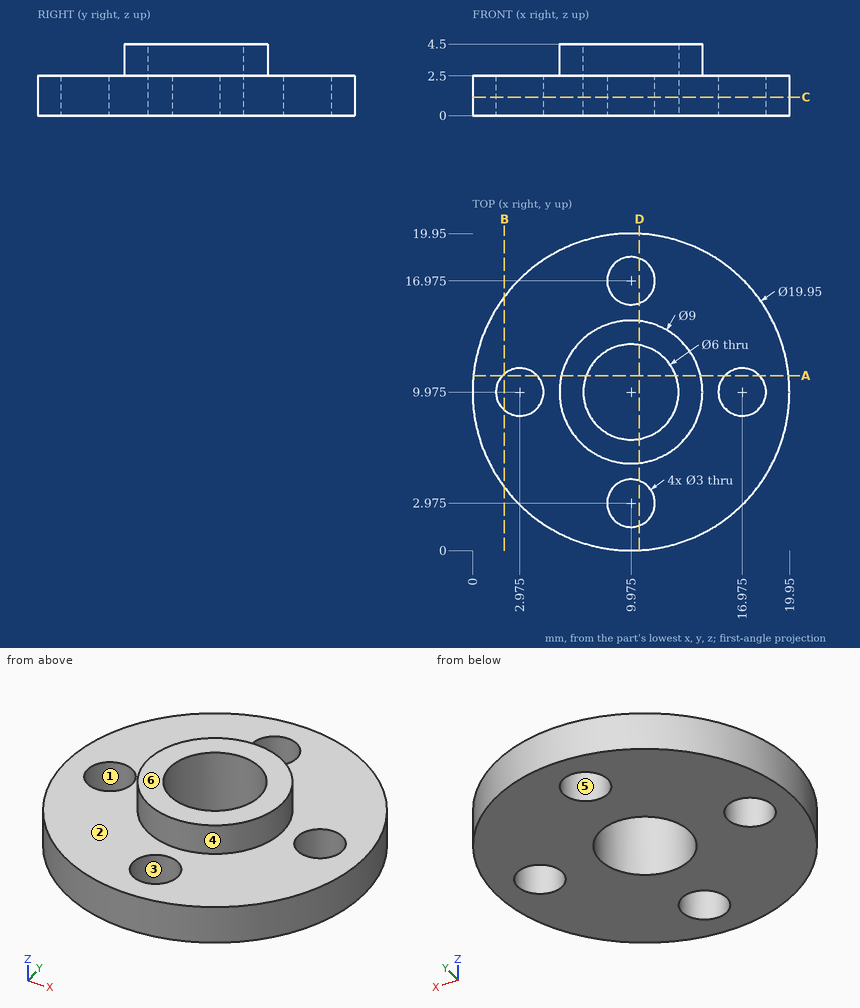
For this review, use the dimensioned drawing (mm, ordinates from the lowest corner) and the shaded views. A direction names the side the tool comes from. Coordinates: 2 decimals unless noted, no trailing zeros. Loops run counter-clockwise (first coordinate to the right, second up) from the corner with the lowest first, then second, coordinate; pieces in that order, holes last.
1. For line 1 (Y direction, x = 10.5, z = 2.15); line 2 (X direction, y = 11, z = 1.4); line 3 (Y direction, x = 9, z = 1.65), list the stretches that pass through material, from the lowest coordinate up.
2. Add section D-D, the plane x = 10.5. Give the boundary of the cut face in (y, z), then the cut area to 3 significant figures.
3. Add section B-B, the plane x = 2. Give the boundary of the cut face in (y, z).
4. Add section A-A, the plane y = 11. Give the boundary of the cut face in (x, z).
5. Mouldability with a two-part tool opening along X and no side actions: class the marked faces 3, 4, 5 and 6 as +X half, -X half, draft (parallel to the pull), parting line (faces both ways), or undercut.
6. Insertion check: P1, Ø1, axis at x = 7, z = 2, coming from the +Y side; P2, Ø4, axis at x = 16.975, y = 9.975, coming from the +Z side; P3, Ø2, axis at y = 8.5, z = 0.5, coming from the +X side; P4, Ø2.5, axis at x = 9.975, y = 2.975, coming from the +Z side. Each pin has a flat end and moves straight along its axis. Give the tip position at first contact, or say it passes through.
7. Add section C-C, the plane z = 1.15. Give the boundary of the cut face in (x, y) (3 decimals), then the cut area to 3 significant figures.
8. For the marked faces 1 and 2, list the 3-axis set-ups (+Z, -Z, +X, -X, +Y, -Y) from which the entire face can be reached by the end or side of a thin tool; tool diameter is ignored.
Result:
1. line 1: y = 0.01 to 1.57, 4.38 to 7.02, 12.93 to 15.57, 18.38 to 19.94
1. line 2: x = 0.05 to 1.88, 4.07 to 7.16, 12.79 to 15.88, 18.07 to 19.9
1. line 3: y = 0.05 to 1.84, 4.11 to 7.14, 12.81 to 15.84, 18.11 to 19.9
2. outline: (0.01, 0) - (1.57, 0) - (1.57, 2.5) - (0.01, 2.5) - close; (4.38, 0) - (7.02, 0) - (7.02, 4.5) - (5.51, 4.5) - (5.51, 2.5) - (4.38, 2.5) - close; (12.93, 0) - (15.57, 0) - (15.57, 2.5) - (14.44, 2.5) - (14.44, 4.5) - (12.93, 4.5) - close; (18.38, 0) - (19.94, 0) - (19.94, 2.5) - (18.38, 2.5) - close
2. area: 27.0 mm2
3. outline: (3.98, 0) - (8.84, 0) - (8.84, 2.5) - (3.98, 2.5) - close; (11.11, 0) - (15.97, 0) - (15.97, 2.5) - (11.11, 2.5) - close
4. outline: (0.05, 0) - (1.88, 0) - (1.88, 2.5) - (0.05, 2.5) - close; (4.07, 0) - (7.16, 0) - (7.16, 4.5) - (5.59, 4.5) - (5.59, 2.5) - (4.07, 2.5) - close; (12.79, 0) - (15.88, 0) - (15.88, 2.5) - (14.36, 2.5) - (14.36, 4.5) - (12.79, 4.5) - close; (18.07, 0) - (19.9, 0) - (19.9, 2.5) - (18.07, 2.5) - close
5. face 3: undercut
5. face 4: parting line
5. face 5: undercut
5. face 6: draft
6. P1: stops at y = 19.64
6. P2: stops at z = 2.5
6. P3: stops at x = 19.94
6. P4: passes through
7. outline: circle Ø19.95 at (9.975, 9.975); hole circle Ø3 at (2.975, 9.975); hole circle Ø6 at (9.975, 9.975); hole circle Ø3 at (9.975, 2.975); hole circle Ø3 at (9.975, 16.975); hole circle Ø3 at (16.975, 9.975)
7. area: 256 mm2
8. face 1: +Z, -Z
8. face 2: +Z
